```python
from build123d import *

# Parameters (mm, degrees)
SKETCH1_W           = 53.975
SKETCH1_H           = 25.4
BOSS_EXTRUDE1_DEPTH = 9.525
SKETCH2_W           = 42
SKETCH2_H           = 21
CUT_EXTRUDE1_DEPTH  = 6.725
FILLET1_R           = 1
SKETCH3_R           = 3.175
BOSS_EXTRUDE2_DEPTH = 14.2875
SKETCH4_R           = 1.5875
CUT_EXTRUDE2_DEPTH  = 9.525
FILLET2_R           = 6.35
SKETCH5_W           = 5.9875
SKETCH5_H           = 7.9375
CUT_EXTRUDE3_DEPTH  = 6.725
FILLET3_R           = 1.5875


with BuildPart() as part:
    # Sketch1 → Boss-Extrude1 (new body)
    with BuildSketch(Plane(origin=(0, 0, 0), x_dir=(1, 0, 0), z_dir=(0, 1, 0))):
        with Locations((26.9875, 12.7)):
            Rectangle(SKETCH1_W, SKETCH1_H)
    extrude(amount=BOSS_EXTRUDE1_DEPTH)

    # Sketch2 → Cut-Extrude1 (cut)
    with BuildSketch(Plane(origin=(0, 9.525, 0), x_dir=(1, 0, 0), z_dir=(0, 1, 0))):
        with Locations((26.9875, 12.7)):
            Rectangle(SKETCH2_W, SKETCH2_H)
    extrude(amount=-CUT_EXTRUDE1_DEPTH, mode=Mode.SUBTRACT)

    # Fillet1
    fillet1_edges = [part.edges().sort_by_distance(p)[0] for p in [
        (5.9875, 6.1625, -2.2),
        (5.9875, 6.1625, -23.2),
        (47.9875, 6.1625, -23.2),
        (47.9875, 6.1625, -2.2),
    ]]
    fillet(fillet1_edges, radius=FILLET1_R)

    # Sketch3 → Boss-Extrude2 (add)
    with BuildSketch(Plane.XZ):
        with Locations((37.4875, -12.7)):
            Circle(SKETCH3_R)
    extrude(amount=BOSS_EXTRUDE2_DEPTH)

    # Sketch4 → Cut-Extrude2 (cut)
    with BuildSketch(Plane(origin=(0, 9.525, 0), x_dir=(1, 0, 0), z_dir=(0, 1, 0))):
        with Locations((3.175, 20.6375)):
            Circle(SKETCH4_R)
        with Locations((3.175, 4.7625)):
            Circle(SKETCH4_R)
        with Locations((50.8, 20.6375)):
            Circle(SKETCH4_R)
        with Locations((50.8, 4.7625)):
            Circle(SKETCH4_R)
    extrude(amount=-CUT_EXTRUDE2_DEPTH, mode=Mode.SUBTRACT)

    # Fillet2
    fillet2_edges = [part.edges().sort_by_distance(p)[0] for p in [
        (0, 4.7625, -25.4),
        (53.975, 4.7625, -25.4),
        (53.975, 4.7625, 0),
        (0, 4.7625, 0),
    ]]
    fillet(fillet2_edges, radius=FILLET2_R)

    # Sketch5 → Cut-Extrude3 (cut)
    with BuildSketch(Plane(origin=(0, 9.525, 0), x_dir=(1, 0, 0), z_dir=(0, 1, 0))):
        with Locations((50.98125, 12.7)):
            Rectangle(SKETCH5_W, SKETCH5_H)
    extrude(amount=-CUT_EXTRUDE3_DEPTH, mode=Mode.SUBTRACT)

    # Fillet3
    fillet3_edges = [part.edges().sort_by_distance(p)[0] for p in [
        (53.975, 6.1625, -8.73125),
        (47.9875, 6.1625, -8.73125),
        (47.9875, 6.1625, -16.66875),
        (53.975, 6.1625, -16.66875),
    ]]
    fillet(fillet3_edges, radius=FILLET3_R)


solid = part.part
```
For this review, take the finished solid that the model builds, in its own axes (mm). A direction names the side the tool comes from. Coordinates: 2 decimals unless noted, no trailing zeros. Write each loop counter-clockwise with the first axis right and the second up, starting at its lowest first coordinate (ties: lowest second). Pieces come first, ordered by that corner, then holes. Notation, with made-up numbers: (11, 52.5) - (57, 52.5) arc R27 ccw to (57, 68.5) - close; hole circle Ø7 at (82, 21.25). An arc over 180 degrees is marked (long way). Answer in a Markdown table with one row per item. Add a question column.
Q1. We need section C-C, the plane z = -12.7. State the section outline as (x, y) points (1 decimal).
Q2. Draft analysis for pull direction X (two halves, no side actions). For faces 1 (the flat face through (27, 5, -25.4)), 2 (the cylindrical face through (53.522, 6.115, -17.146)), 3 (the cylindrical face through (2.005, 4.829, -21.71)), state which applies: +X half, -X half, draft (parallel to the pull), parting line (faces both ways), or undercut.
Q3. For probe 1 along Z at (x, y) = (13, 7); probe 2 along Y at (x, z) = (4.5, -18) (3 decimals); probe 3 along Z at (x, y) = (50, 5.5), list the stretches that pass through material, from the lowest coordinate up.
Q4. For P1, Ø3.5, axis at y = 6.5, z = -9.5, coming from the +X side; P2, Ø4, axis at x = 27, z = -14, coming from the +Y side; P3, Ø3, axis at x = 3.18, z = -4.76, coming from the +Y side (1 decimal); P4, Ø4, axis at x = 3.18, z = -20.64, coming from the -Y side, all flat-tipped, find the tip position at first contact; note any pin that passes through.
Q5. We need section A-A, the plane x = 50.8. State the section outline as (y, z) points (3 decimals).
Q6. We need section B-B, the plane y = 2.25. Count the separate pieces of the cut face and the enclosed holes in it, and give its area (3 significant figures).
Q7. We need section D-D, the plane x = 25. State the section outline as (y, z) points (3 decimals).
Q8. Tool access review of faces 4 (the flat face through (27, 5, 0)), 5 (the cylindrical face through (48.44, 6.115, -8.254)): name each direction out of +Z, -Z, +X, -X, +Y, -Y from which nothing blocks a thin tool from reaching the whole face with its end or side.
Answer list:
| question | item | result |
|---|---|---|
| 1 | outline | (0, 0) - (34.3, 0) - (34.3, -14.3) - (40.7, -14.3) - (40.7, 0) - (54, 0) - (54, 2.8) - (6, 2.8) - (6, 9.5) - (0, 9.5) - close |
| 2 | face 1 | draft |
| 2 | face 2 | +X half |
| 2 | face 3 | undercut |
| 3 | probe 1 | z = -25.4 to -23.2, -2.2 to 0 |
| 3 | probe 2 | y = 0 to 9.525 |
| 3 | probe 3 | z = -24.94 to -22.01, -19.27 to -16.67, -8.73 to -6.13, -3.39 to -0.46 |
| 4 | P1 | stops at x = 53.85 |
| 4 | P2 | stops at y = 2.8 |
| 4 | P3 | passes through |
| 4 | P4 | stops at y = 0 |
| 5 | outline | (0, -24.549) - (9.525, -24.549) - (9.525, -22.225) - (0, -22.225) - close; (0, -19.05) - (9.525, -19.05) - (9.525, -16.669) - (2.8, -16.669) - (2.8, -8.731) - (9.525, -8.731) - (9.525, -6.35) - (0, -6.35) - close; (0, -3.175) - (9.525, -3.175) - (9.525, -0.851) - (0, -0.851) - close |
| 6 | separate pieces | 1 |
| 6 | enclosed holes | 4 |
| 6 | area | 1,300 mm2 |
| 7 | outline | (0, -25.4) - (9.525, -25.4) - (9.525, -23.2) - (2.8, -23.2) - (2.8, -2.2) - (9.525, -2.2) - (9.525, 0) - (0, 0) - close |
| 8 | face 4 | +Z, +X, -X, +Y, -Y |
| 8 | face 5 | +Y |
